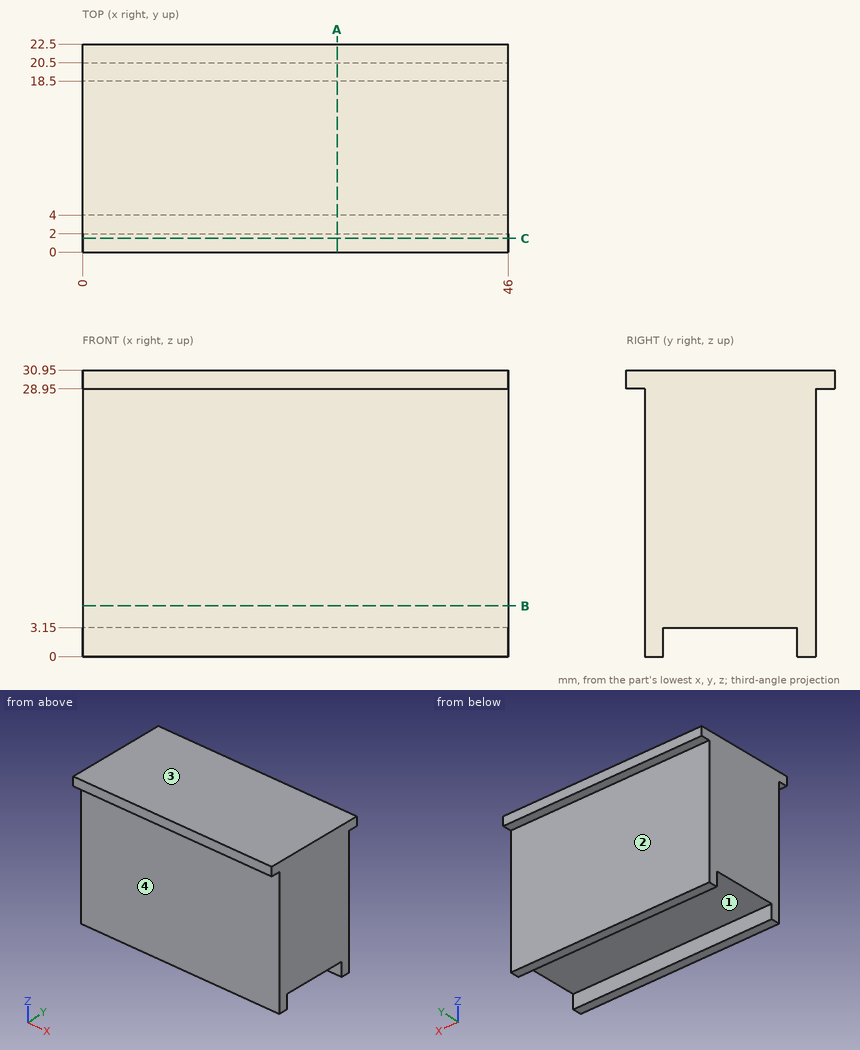
For this review, use the dimensioned drawing (mm, ordinates from the lowest corner) and the shaded views. Round coordinates to 2 decimals unless told otherwise and drop trailing zeros. Order: outer loops, then holes, each group sorted by start corner. A loop starts at its lowest first (then second) coordinate and runs counter-clockwise, first axis right, second up. Notation, with made-up numbers: M 1,79.5 L 9,79.5 A32 cw 9,111.5 Z; hole C 10.25,9 d8. An arc over 180 degrees is marked long. Write each question's results on one line, items separated by ' | '. Start each with the question number.
1. Clearance check with flat-ended pins moving along their axes: pin 1 Ø2 at (x, y) = (25, 21) entering from -Z; pin 2 Ø5 at (x, z) = (7, 22.5) entering from +Y; pin 3 Ø1.6 at (x, y) = (19, 1) entering from -Z; pin 4 Ø8.5 at (x, z) = (14.5, 9.5) entering from -Y. State where each tip first meets the part, or that it passes through.
2. Draft analysis for pull direction Y (two halves, no side actions). For the marked faces 1, 2, 3 and 4, state which applies: pulls with the +Y half, pulls with the -Y half, needs draft (parallel to the pull), parting line crosses it, or undercut.
3. Add section A-A (x = 27.5). State the section outline as (y, z) points.
4. To check wall thickness, follow L1, parallel to Z at x = 11.5, y = 6.75; L2, parallel to Z at x = 31, y = 1; L3, parallel to Y at x = 44, z = 12. State the ranges of each line that lie inside material, in increasing order. Write a range as [from, to].
5. Add section C-C (y = 1.5). State the section outline as (x, z) points.
6. Add section B-B (z = 5.5). State the section outline as (x, y) points.
Output values:
1) pin 1: z = 0 | pin 2: y = 20.5 | pin 3: z = 28.95 | pin 4: y = 2
2) face 1: undercut | face 2: pulls with the +Y half | face 3: needs draft | face 4: pulls with the -Y half
3) outline: M 0,28.95 L 2,28.95 L 2,0 L 4,0 L 4,3.15 L 18.5,3.15 L 18.5,0 L 20.5,0 L 20.5,28.95 L 22.5,28.95 L 22.5,30.95 L 0,30.95 Z
4) L1: [3.15, 30.95] | L2: [28.95, 30.95] | L3: [2, 20.5]
5) outline: M 0,28.95 L 46,28.95 L 46,30.95 L 0,30.95 Z
6) outline: M 0,2 L 46,2 L 46,20.5 L 0,20.5 Z
